```python
from build123d import *

# Parameters (mm, degrees)
F0_R     = 29.735
F1_DEPTH = 6.4
F2_R     = 9.75
F3_DEPTH = 3.9
F4_W     = 17
F4_H     = 14.5
F5_DEPTH = 2


with BuildPart() as f1:
    # F0 (on Top) → F1 (new body)
    with BuildSketch(Plane.XY):
        Circle(F0_R)
    extrude(amount=F1_DEPTH)

    # F2 (on face) → F3 (cut)
    with BuildSketch(Plane.XY.offset(6.4)):
        with Locations((0, 12.815)):
            Circle(F2_R)
        with Locations((0, -15.835)):
            Circle(F2_R)
    extrude(amount=-F3_DEPTH, mode=Mode.SUBTRACT)

    # F4 (on face) → F5 (cut)
    with BuildSketch(Plane(origin=(0, 0, 0), x_dir=(1, 0, 0), z_dir=(0, 0, -1))):
        Rectangle(F4_W, F4_H)
    extrude(amount=-F5_DEPTH, mode=Mode.SUBTRACT)


solid = f1.part
```
Input: part model. Units: mm. Frame: model coordinates. A direction names the side the tool comes from. Round coordinates to 2 decimals unless told otherwise and drop trailing zeros. Loops run counter-clockwise (first coordinate to the right, second up) from the corner with the lowest first, then second, coordinate; pieces in that order, holes last. Notation, with made-up numbers: M 29,52 L 72,52 A19 cw 72,56 Z; hole C 25.25,-16 d11. An arc over 180 degrees is marked long. Answer in a Markdown table with one row per item. Add a question column.
1. Section D-D (y = -18.5). Output: boundary loops of the cut face in (x, z), and give its area (3 significant figures).
2. Mould query, pull axis Y, two halves, no side actions, for faces 4 (the face through (-6.446, -29.028, 3.155)), 5 (the face through (0, 0, 6.4)), 6 (the face through (4.499, -24.485, 4.477)), 7 (the face through (-8.5, 0, 1)). Classes: released by +Y, released by -Y, zero draft, split by the parting line, or undercut.
3. Section A-A (z = 1). Output: boundary loops of the cut face in (x, y) (3 decimals).
4. Section B-B (x = 0). Output: boundary loops of the cut face in (y, z) (3 decimals).
5. Section C-C (y = -1). Output: boundary loops of the cut face in (x, z), and give its area (3 significant figures).
6. Contact query for flat-ended pins moving along their axis: pin 1 (2 mm diameter, centred on y = -2, z = 1, fed in from +X); pin 2 (1 mm diameter, centred on x = -23, z = 2, fed in from +Y); pin 3 (3 mm diameter, centred on x = -6, y = 10.5, fed in from +Z). Output: stop coordinate, or through.
7. Set-up query: faces 1 (the face through (0, 0, 2)), 2 (the face through (0, 13, 2.5)), 3 (the face through (0, -13, 0)). Return all of +Z, -Z, +X, -X, +Y, -Y with unobstructed straight access to the full face (end or side cutting, diameter ignored); none if empty.
8. Ray query, probe 1 along Y at (x, z) = (0, 3.6) (3 decimals); probe 2 along X at (y, z) = (0.5, 1.75); probe 3 along Y at (x, z) = (-5.5, 3.5). Return the intervals inside material, ascending.
Values follow:
| question | item | result |
|---|---|---|
| 1 | outline | M -23.28,0 L 23.28,0 L 23.28,6.4 L 9.38,6.4 L 9.38,2.5 L -9.38,2.5 L -9.38,6.4 L -23.28,6.4 Z |
| 1 | area | 225 mm^2 |
| 2 | face 4 | split by the parting line |
| 2 | face 5 | zero draft |
| 2 | face 6 | undercut |
| 2 | face 7 | undercut |
| 3 | outline | C 0,0 d59.47; hole M -8.5,-7.25 L 8.5,-7.25 L 8.5,7.25 L -8.5,7.25 Z |
| 4 | outline | M -29.735,0 L -7.25,0 L -7.25,2 L 7.25,2 L 7.25,0 L 29.735,0 L 29.735,6.4 L 22.565,6.4 L 22.565,2.5 L 3.065,2.5 L 3.065,6.4 L -6.085,6.4 L -6.085,2.5 L -25.585,2.5 L -25.585,6.4 L -29.735,6.4 Z |
| 5 | outline | M -29.72,0 L -8.5,0 L -8.5,2 L 8.5,2 L 8.5,0 L 29.72,0 L 29.72,6.4 L -29.72,6.4 Z |
| 5 | area | 346 mm^2 |
| 6 | pin 1 | x = 29.72 |
| 6 | pin 2 | y = 19.44 |
| 6 | pin 3 | z = 2.5 |
| 7 | face 1 | -Z |
| 7 | face 2 | +Z |
| 7 | face 3 | -Z, +X, -X, +Y, -Y |
| 8 | probe 1 | -29.735 to -25.585, -6.085 to 3.065, 22.565 to 29.735 |
| 8 | probe 2 | -29.73 to -8.5, 8.5 to 29.73 |
| 8 | probe 3 | -29.22 to -23.89, -7.78 to 4.76, 20.87 to 29.22 |
